CAD build for the part. Positions are in the model's coordinates, mm. Coordinates: 2 decimals unless noted, no trailing zeros. Loops run counter-clockwise (first coordinate to the right, second up) from the corner with the lowest first, then second, coordinate; pieces in that order, holes last.
1) Pin check, flat tip, straight feed: pin 1 Ø11.5 at (x, y) = (-114, -64) entering from +Z. Stop position of the tip, or through.
2) Wall check: line 1 along Y through (x, z) = (88.9, 18.75); line 2 along Y through (x, z) = (-114.3, 16.5). Give the ranges that are in metal, low to high.
3) Saw through at B-B, the plane z = 21.5. Give the number of separate pieces and of enclosed holes in the cut face, and give its area (3 significant figures).
4) Saw through at A-A, the plane x = -114.3. Write the cut outline in (y, z), and give its area (3 significant figures).
```python
from build123d import *

# Parameters (mm, degrees)
F0_W           = 254
F0_H           = 152.4
F1_DEPTH       = 25.4
F3_D           = 9.525
F3_CBORE_D     = 14.2875
F3_CBORE_DEPTH = 12.7
F5_D           = 7.9375


# Not quite as in the source:
# - a length typed as a fraction of an inch, garbled in the dataset ("3 / 203.2 mm" for 3/8 in), is restored


with BuildPart() as f1:
    # F0 (on Top) → F1 (new body)
    with BuildSketch(Plane.XY):
        Rectangle(F0_W, F0_H)
    extrude(amount=F1_DEPTH)

    # F3 (through all)
    with Locations(Plane.XY.offset(25.4)):
        with Locations((-114.3, 63.5), (-114.3, -63.5), (114.3, 63.5), (114.3, -63.5)):
            CounterBoreHole(F3_D / 2, F3_CBORE_D / 2, F3_CBORE_DEPTH)

    # F5 (through all)
    with Locations(Plane.XY.offset(25.4)):
        with Locations((-88.9, 63.5), (0, 63.5), (88.9, 63.5), (88.9, -63.5), (0, -63.5), (-88.9, -63.5)):
            Hole(F5_D / 2)


solid = f1.part
```
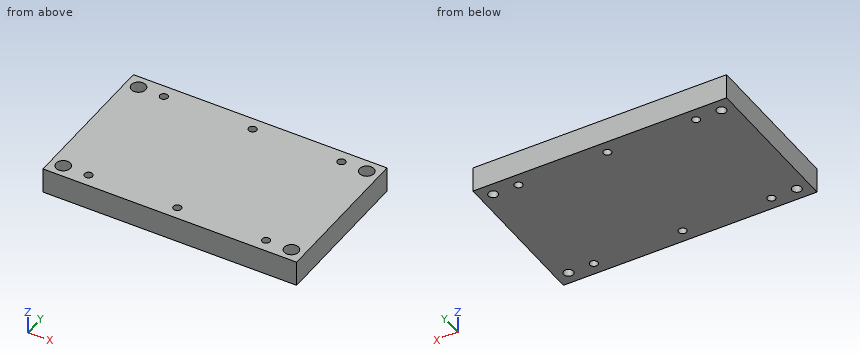
Data:
1. pin 1: stops at z = 12.7
2. line 1: y = -76.2 to -67.47, -59.53 to 59.53, 67.47 to 76.2
2. line 2: y = -76.2 to -70.64, -56.36 to 56.36, 70.64 to 76.2
3. separate pieces: 1
3. enclosed holes: 10
3. area: 37,800 mm2
4. outline: (-76.2, 0) - (-68.26, 0) - (-68.26, 12.7) - (-70.64, 12.7) - (-70.64, 25.4) - (-76.2, 25.4) - close; (-58.74, 0) - (58.74, 0) - (58.74, 12.7) - (56.36, 12.7) - (56.36, 25.4) - (-56.36, 25.4) - (-56.36, 12.7) - (-58.74, 12.7) - close; (68.26, 0) - (76.2, 0) - (76.2, 25.4) - (70.64, 25.4) - (70.64, 12.7) - (68.26, 12.7) - close
4. area: 3,270 mm2
